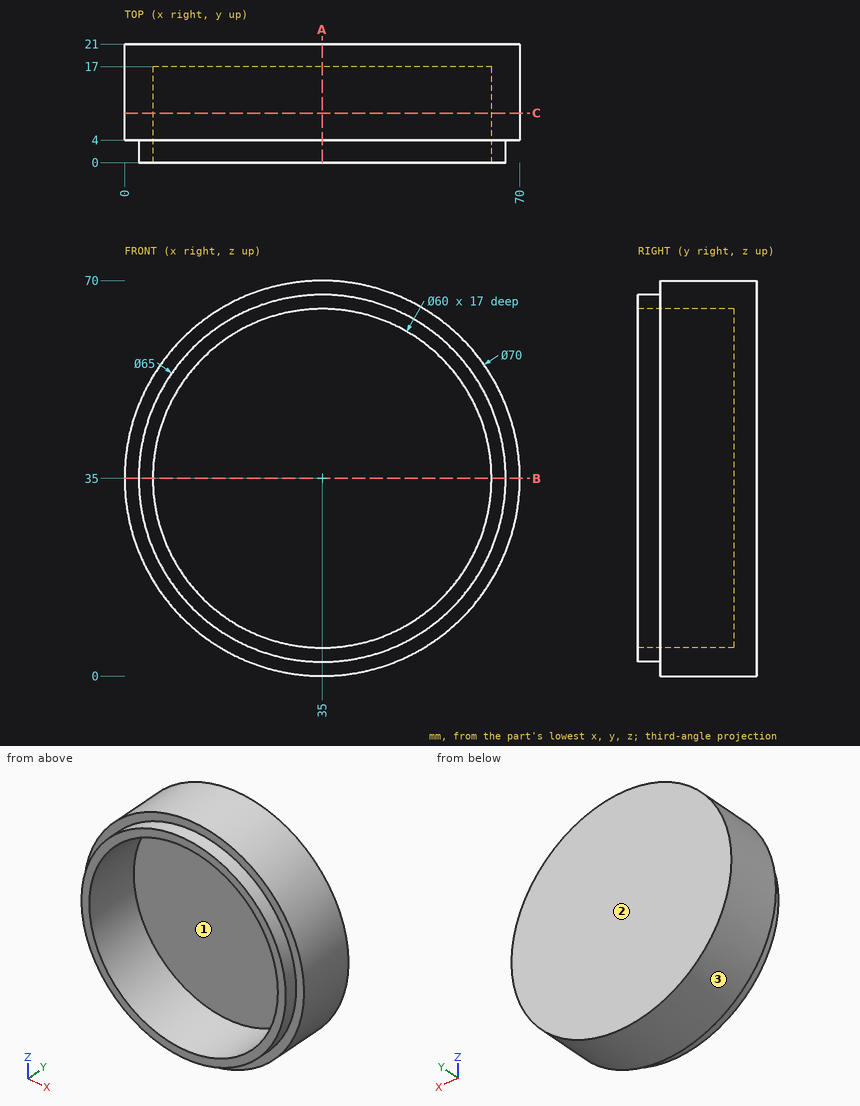
Can you work these out from the drawing? Everything is in mm from the part's minimum corner. Round coordinates to 2 decimals unless told otherwise and drop trailing zeros. Write each loop counter-clockwise with the first axis right and the second up, starting at its lowest first coordinate (ties: lowest second). Pieces come first, ordered by that corner, then holes.
1. Suppose I cut it at B-B (z = 35). List the corners of the cut face in (x, y) for me, and give its area (3 significant figures).
2. Suppose I cut it at A-A (x = 35). List the corners of the cut face in (y, z) for me.
3. If we mould it in two halves opening along X, with no side actions, what happens to the marked faces 1, 2 and 3? For each: released by +X, released by -X, zero draft, split by the parting line, or undercut.
4. Suppose I cut it at C-C (y = 8.75). List the corners of the cut face in (x, z) for me.
5. I need wall thicknesses on L1, parallel to Z at x = 35, y = 5.5; L2, parallel to Z at x = 34.5, y = 17.5; L3, parallel to Y at x = 54.5, z = 19.5. Which ranges of each line are inside material? Lowest first, please.
6. Will these pins go through, and if not, where does the flat tip stop? pin 1 Ø8 at (x, y) = (46.5, 10.5) entering from +Z; pin 2 Ø1 at (x, y) = (15.5, 17.5) entering from +Z; pin 3 Ø5 at (x, z) = (48, 27) entering from -Y.
Answer sheet:
1. outline: (0, 4) - (2.5, 4) - (2.5, 0) - (5, 0) - (5, 17) - (65, 17) - (65, 0) - (67.5, 0) - (67.5, 4) - (70, 4) - (70, 21) - (0, 21) - close
1. area: 430 mm2
2. outline: (0, 2.5) - (4, 2.5) - (4, 0) - (21, 0) - (21, 70) - (4, 70) - (4, 67.5) - (0, 67.5) - (0, 65) - (17, 65) - (17, 5) - (0, 5) - close
3. face 1: undercut
3. face 2: zero draft
3. face 3: split by the parting line
4. outline: circle Ø70 at (35, 35); hole circle Ø60 at (35, 35)
5. L1: z = 0 to 5, 65 to 70
5. L2: z = 0 to 70
5. L3: y = 17 to 21
6. pin 1: stops at z = 69.19
6. pin 2: stops at z = 64.39
6. pin 3: stops at y = 17
